Answer from the drawing. Dimensions are ordinates in mm from the lowest x, y and z of the part. A direction names the side the tool comes from. Coordinates: 2 decimals unless noted, no trailing zeros. Write each loop counter-clockwise with the first axis right and the second up, starting at its lowest first coordinate (ties: lowest second). Pieces come first, ordered by that corner, then holes. Notation, with made-up numbers: (-1.5, 59) -> (32.5, 59) arc R23 ccw to (32.5, 92) -> close; hole circle Ø6 at (-14.75, 88). An arc over 180 degrees is marked (long way). One line per item, written item: value. Start each with the question number.
1. For the marked faces 1, 2 and 3, determine the directions among +Z, -Z, +X, -X, +Y, -Y from which every point of the face is accessible in a straight line to the end or side of a thin tool.
2. Given P1, Ø19.5, axis at x = 12, z = 25, coming from the -Y side; P2, Ø2.5, axis at y = 2.5, z = 25, coming from the +X side; P3, Ø1.5, axis at x = 24.5, y = 2.5, coming from the +Z side; P4, Ø1.5, axis at y = 1.5, z = 25.5, coming from the -X side, each flat-ended and moving along its own axis, determine where each tip first touches the part or whether it passes through.
3. Find section A-A, the plane y = 6.25. Write down the section's boundary in (x, z), and give its area (3 significant figures).
4. Consider line 1 along X through (y, z) = (4.5, 25.5); line 2 along Y through (x, z) = (2, 29); line 3 along Z through (x, y) = (28.5, 4.5). Determine where each line is inside the solid, lowest interval first.
5. Find section D-D, the plane x = 11. Write down the section's boundary in (y, z).
6. Find section B-B, the plane x = 19.3. Write down the section's boundary in (y, z), and give its area (3 significant figures).
7. Find section C-C, the plane z = 37. Write down the section's boundary in (x, y).
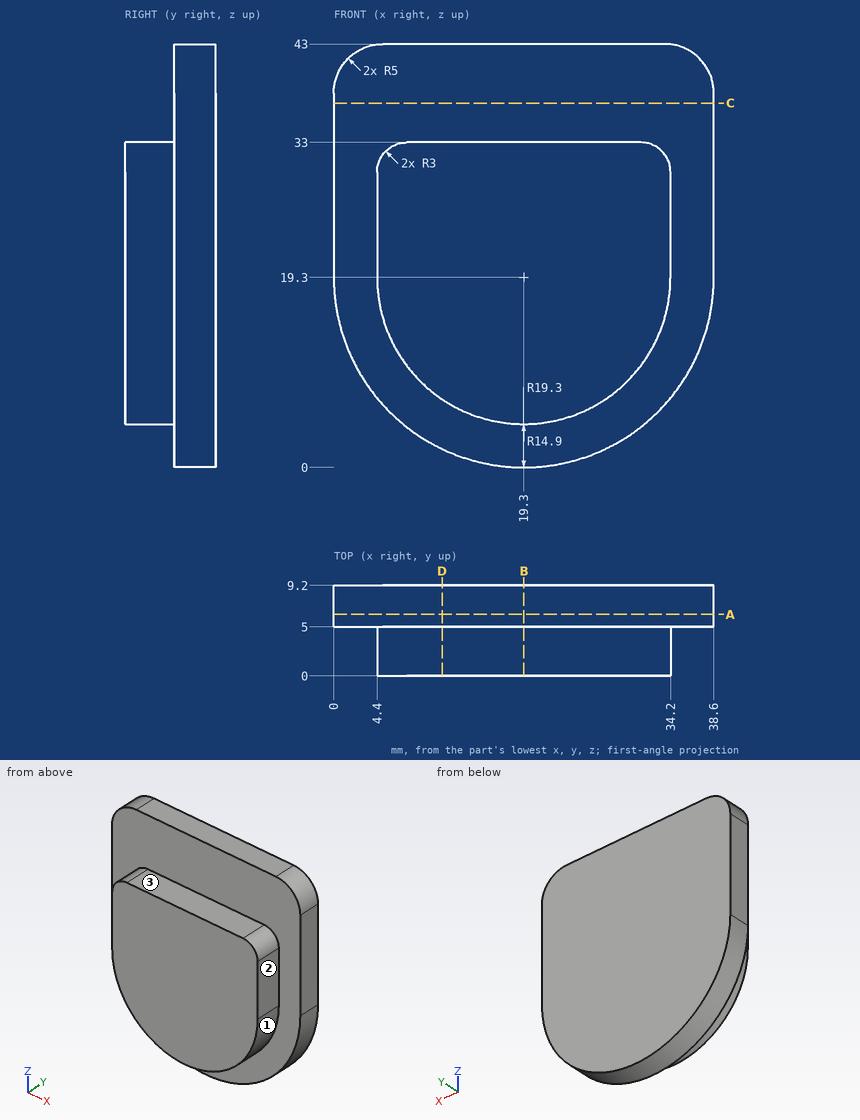
Answer block:
1. face 1: -Z, -Y
1. face 2: +Z, -Z, +X, -Y
1. face 3: +Z, +X, -X, -Y
2. P1: stops at y = 0
2. P2: stops at x = 34.2
2. P3: stops at z = 33
2. P4: stops at x = 4.4
3. outline: (0, 19.3) arc R19.3 ccw to (38.6, 19.3) -> (38.6, 38) arc R5 ccw to (33.6, 43) -> (5, 43) arc R5 ccw to (0, 38) -> close
3. area: 1,490 mm2
4. line 1: x = 4.4 to 34.2
4. line 2: y = 5 to 9.2
4. line 3: z = 7.58 to 33
5. outline: (0, 6.93) -> (5, 6.93) -> (5, 1.88) -> (9.2, 1.88) -> (9.2, 43) -> (5, 43) -> (5, 33) -> (0, 33) -> close
6. outline: (0, 4.4) -> (5, 4.4) -> (5, 0) -> (9.2, 0) -> (9.2, 43) -> (5, 43) -> (5, 33) -> (0, 33) -> close
6. area: 324 mm2
7. outline: (0, 5) -> (38.6, 5) -> (38.6, 9.2) -> (0, 9.2) -> close
